```python
from build123d import *

# Parameters (mm, degrees)
CUT_EXTRUDE1_REACH = 21.404
SKETCH2_R          = 1.5


with BuildPart() as part:
    # Sketch1 → Revolve1 (revolve)
    with BuildSketch(Plane(origin=(0, 0, 0), x_dir=(0, 0, -1), z_dir=(1, 0, 0)), mode=Mode.PRIVATE) as revolve1_sk:
        Polygon((-5, 0), (-12.5, 0), (-12.5, 2), (-7, 2), (-7, 10), (-5, 10), align=None)
    revolve(revolve1_sk.sketch.rotate(Axis((0, -0.941879477, 0), (0, 1, 0)), 180), axis=Axis((0, -0.941879477, 0), (0, 1, 0)))

    # Sketch2 → Cut-Extrude1 (cut, up to next)
    with BuildSketch(Plane(origin=(0, 2, 0), x_dir=(1, 0, 0), z_dir=(0, 1, 0)), mode=Mode.PRIVATE) as cut_extrude1_sk1:
        with Locations(Location((0, 10, 0), (0, 0, 270))):
            Circle(SKETCH2_R)
    cut_extrude1_tool1 = extrude(cut_extrude1_sk1.sketch, amount=-CUT_EXTRUDE1_REACH, mode=Mode.PRIVATE) & part.part
    # Sketch2 → Cut-Extrude1 (cut, up to next)
    with BuildSketch(Plane(origin=(0, 2, 0), x_dir=(1, 0, 0), z_dir=(0, 1, 0)), mode=Mode.PRIVATE) as cut_extrude1_sk2:
        with Locations(Location((10, 0, 0), (0, 0, 270))):
            Circle(SKETCH2_R)
    cut_extrude1_tool2 = extrude(cut_extrude1_sk2.sketch, amount=-CUT_EXTRUDE1_REACH, mode=Mode.PRIVATE) & part.part
    # Sketch2 → Cut-Extrude1 (cut, up to next)
    with BuildSketch(Plane(origin=(0, 2, 0), x_dir=(1, 0, 0), z_dir=(0, 1, 0)), mode=Mode.PRIVATE) as cut_extrude1_sk3:
        with Locations(Location((0, -10, 0), (0, 0, 270))):
            Circle(SKETCH2_R)
    cut_extrude1_tool3 = extrude(cut_extrude1_sk3.sketch, amount=-CUT_EXTRUDE1_REACH, mode=Mode.PRIVATE) & part.part
    # Sketch2 → Cut-Extrude1 (cut, up to next)
    with BuildSketch(Plane(origin=(0, 2, 0), x_dir=(1, 0, 0), z_dir=(0, 1, 0)), mode=Mode.PRIVATE) as cut_extrude1_sk4:
        with Locations(Location((-10, 0, 0), (0, 0, 270))):
            Circle(SKETCH2_R)
    cut_extrude1_tool4 = extrude(cut_extrude1_sk4.sketch, amount=-CUT_EXTRUDE1_REACH, mode=Mode.PRIVATE) & part.part
    add(cut_extrude1_tool1.solids().sort_by_distance((0, 2, -10))[0], mode=Mode.SUBTRACT)
    add(cut_extrude1_tool2.solids().sort_by_distance((10, 2, 0))[0], mode=Mode.SUBTRACT)
    add(cut_extrude1_tool3.solids().sort_by_distance((0, 2, 10))[0], mode=Mode.SUBTRACT)
    add(cut_extrude1_tool4.solids().sort_by_distance((-10, 2, 0))[0], mode=Mode.SUBTRACT)


solid = part.part
```
Geometry: final body of the model. Coordinates: model frame, mm. Coordinates: 2 decimals unless noted, no trailing zeros. Order: outer loops, then holes, each group sorted by start corner. A loop starts at its lowest first (then second) coordinate and runs counter-clockwise, first axis right, second up.
Item 1: Contact query for flat-ended pins moving along their axis: P1, Ø1, axis at x = 7, z = 4, coming from the +Y side; P2, Ø2.5, axis at x = -10, z = 0, coming from the -Y side; P3, Ø2, axis at x = -1, z = 4, coming from the -Y side; P4, Ø5, axis at x = -6, y = 5, coming from the -Z side. Output: stop coordinate, or through.
Answer:
P1: stops at y = 2
P2: passes through
P3: stops at y = 0
P4: stops at z = -6.06
Item 2: Section query D-D (x = 0). Output: boundary loops of the cut face in (y, z).
Answer:
outline: (0, -12.5) - (2, -12.5) - (2, -11.5) - (0, -11.5) - close; (0, -8.5) - (2, -8.5) - (2, -7) - (10, -7) - (10, -5) - (0, -5) - close; (0, 5) - (10, 5) - (10, 7) - (2, 7) - (2, 8.5) - (0, 8.5) - close; (0, 11.5) - (2, 11.5) - (2, 12.5) - (0, 12.5) - close
Item 3: Section query A-A (z = 0). Output: boundary loops of the cut face in (x, y).
Answer:
outline: (-12.5, 0) - (-11.5, 0) - (-11.5, 2) - (-12.5, 2) - close; (-8.5, 0) - (-5, 0) - (-5, 10) - (-7, 10) - (-7, 2) - (-8.5, 2) - close; (5, 0) - (8.5, 0) - (8.5, 2) - (7, 2) - (7, 10) - (5, 10) - close; (11.5, 0) - (12.5, 0) - (12.5, 2) - (11.5, 2) - close
Item 4: Section query C-C (z = -10). Output: boundary loops of the cut face in (x, y).
Answer:
outline: (-7.5, 0) - (-1.5, 0) - (-1.5, 2) - (-7.5, 2) - close; (1.5, 0) - (7.5, 0) - (7.5, 2) - (1.5, 2) - close
Item 5: Section query B-B (x = 10). Output: boundary loops of the cut face in (y, z).
Answer:
outline: (0, -7.5) - (2, -7.5) - (2, -1.5) - (0, -1.5) - close; (0, 1.5) - (2, 1.5) - (2, 7.5) - (0, 7.5) - close
Item 6: Material intervals for line 1 along X through (y, z) = (3, 0); line 2 along Y through (x, z) = (8.5, 6.25); line 3 along X through (y, z) = (1.05, -10), sorted ascending.
Answer:
line 1: x = -7 to -5, 5 to 7
line 2: y = 0 to 2
line 3: x = -7.5 to -1.5, 1.5 to 7.5
Item 7: Draft query along X for faces 1 (the face through (5.4, 2, -5.4)), 2 (the face through (-11.464, 1.014, -0.325)), 3 (the face through (2.681, 6.056, -6.466)), 4 (the face through (0, 5, 5)). Return one class per face: released by +X, released by -X, zero draft, split by the parting line, or undercut.
Answer:
face 1: zero draft
face 2: undercut
face 3: split by the parting line
face 4: undercut
